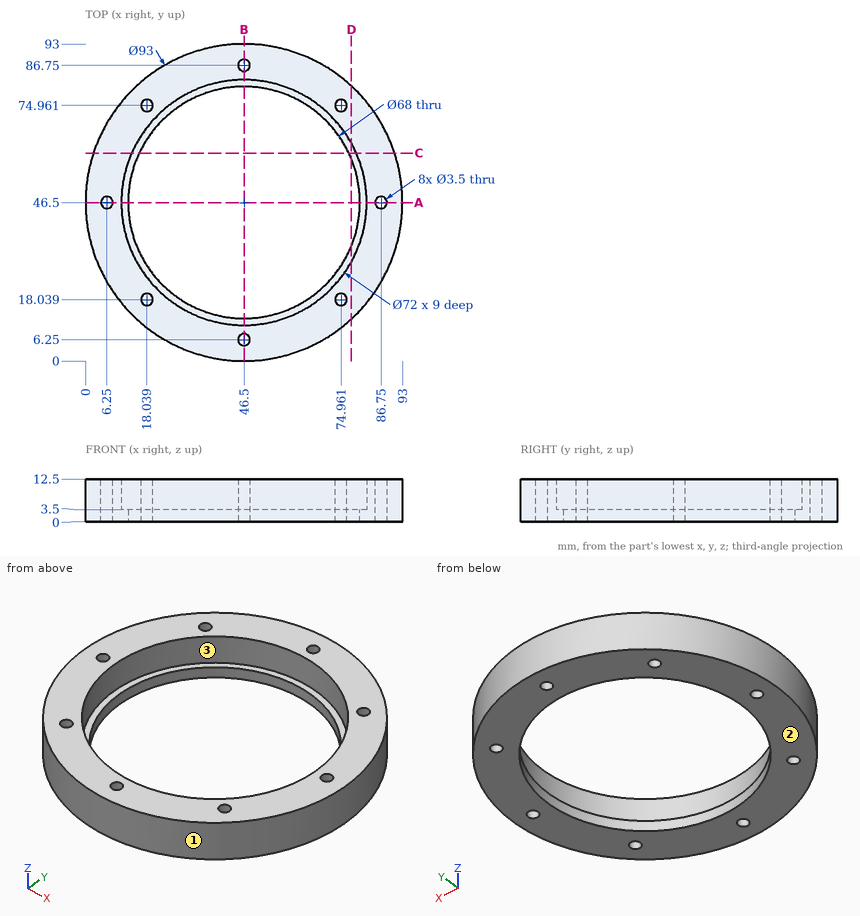
Geometry check sheet. Reference: drawing and pictorial views, mm from the part's lowest x, y, z. Give positions to 0.01 mm unless a question says otherwise; leave off trailing zeros. Loops run counter-clockwise (first coordinate to the right, second up) from the corner with the lowest first, then second, coordinate; pieces in that order, holes last.
1. Section check A-A, the plane y = 46.5. Enter the section's corners in (x, z).
2. Thickness scan on line 1 (X direction, y = 48, z = 4); line 2 (Z direction, x = 19, y = 68); line 3 (Y direction, x = 69.5, z = 1.25). Record the ranges inside material, lowest first.
3. Section check D-D, the plane x = 78. Enter the section's corners in (y, z), then the cut area to 3 significant figures.
4. Mould release check, pull along X, two halves, no side actions. Record for the marked faces 1, 2 and 3: released by +X, released by -X, zero draft, split by the parting line, or undercut.
5. Section check C-C, the plane y = 61. Enter the section's corners in (x, z), then the cut area to 3 significant figures.
6. Go/stop test with flat-tipped pins: pin 1 Ø3 at (y, z) = (57.5, 9.5) entering from -X; pin 2 Ø1 at (x, z) = (31, 2.5) entering from -Y; pin 3 Ø1.5 at (x, z) = (24.5, 3) entering from -Y. Record where each tip stops, or that it passes through.
Geometry says:
1. outline: (0, 0) - (4.5, 0) - (4.5, 12.5) - (0, 12.5) - close; (8, 0) - (12.5, 0) - (12.5, 3.5) - (10.5, 3.5) - (10.5, 12.5) - (8, 12.5) - close; (80.5, 0) - (85, 0) - (85, 12.5) - (82.5, 12.5) - (82.5, 3.5) - (80.5, 3.5) - close; (88.5, 0) - (93, 0) - (93, 12.5) - (88.5, 12.5) - close
2. line 1: x = 0.02 to 5.35, 7.15 to 10.53, 82.47 to 85.85, 87.65 to 92.98
2. line 2: z = 0 to 3.5
2. line 3: y = 6.09 to 21.46, 71.54 to 86.91
3. outline: (12.29, 0) - (33.7, 0) - (33.7, 3.5) - (29.07, 3.5) - (29.07, 12.5) - (12.29, 12.5) - close; (59.3, 0) - (80.71, 0) - (80.71, 12.5) - (63.93, 12.5) - (63.93, 3.5) - (59.3, 3.5) - close
3. area: 452 mm2
4. face 1: split by the parting line
4. face 2: zero draft
4. face 3: undercut
5. outline: (2.32, 0) - (15.75, 0) - (15.75, 3.5) - (13.55, 3.5) - (13.55, 12.5) - (2.32, 12.5) - close; (77.25, 0) - (90.68, 0) - (90.68, 12.5) - (79.45, 12.5) - (79.45, 3.5) - (77.25, 3.5) - close
5. area: 296 mm2
6. pin 1: stops at x = 0.98
6. pin 2: stops at y = 2.49
6. pin 3: stops at y = 5.14
